from build123d import *

# Parameters (mm, degrees)
ESQUISSE1_R        = 2.5
ESQUISSE1_R_2      = 1.5
BOSS_EXTRU_1_DEPTH = 1.5
CONG_1_R           = 4


with BuildPart() as part:
    # Esquisse1 → Boss.-Extru.1 (new body)
    with BuildSketch(Plane.XY):
        Polygon((38, -20), (38, -32.5), (0, -32.5), (0, 32.5), (38, 32.5), (38, 20), (18, 20), (18, -20), align=None)
        with Locations((8, 25)):
            Circle(ESQUISSE1_R, mode=Mode.SUBTRACT)
        with Locations((23, 24)):
            Circle(ESQUISSE1_R_2, mode=Mode.SUBTRACT)
        with Locations(Location((33, 24, 0), (0, 0, 180))):
            Circle(ESQUISSE1_R_2, mode=Mode.SUBTRACT)
        with Locations((33, -24)):
            Circle(ESQUISSE1_R_2, mode=Mode.SUBTRACT)
        with Locations(Location((23, -24, 0), (0, 0, 180))):
            Circle(ESQUISSE1_R_2, mode=Mode.SUBTRACT)
        with Locations(Location((8, -25, 0), (0, 0, 180))):
            Circle(ESQUISSE1_R, mode=Mode.SUBTRACT)
    extrude(amount=BOSS_EXTRU_1_DEPTH)

    # Congé1
    cong_1_edges = [part.edges().sort_by_distance(p)[0] for p in [
        (38, -32.5, 0.75),
        (0, -32.5, 0.75),
        (0, 32.5, 0.75),
        (38, 32.5, 0.75),
    ]]
    fillet(cong_1_edges, radius=CONG_1_R)


solid = part.part
The listing builds one solid part. Answer for the finished solid, in the listing's coordinates (mm). A direction names the side the tool comes from. Coordinates: 2 decimals unless noted, no trailing zeros. Loops run counter-clockwise (first coordinate to the right, second up) from the corner with the lowest first, then second, coordinate; pieces in that order, holes last. Notation, with made-up numbers: (38.25, 63.5) -> (54.25, 63.5) arc R17 cw to (54.25, 79.5) -> close; hole circle Ø5 at (75, 2). An arc over 180 degrees is marked (long way). Write item = value, one per line. Start each with the question number.
1) A cutting plane is placed at A-A (x = 22.5). Give the vertices of the cut face in (y, z).
2) A cutting plane is placed at B-B (z = 0.3). Give the vertices of the cut face in (x, y), then the cut area to 3 significant figures.
3) A tool of negligible diameter and unlimited length cuts with its end or side. For faces 1 (the face through (31.89, -22.99, 0.74)), 2 (the face through (18, 0, 1)), from which of +Z, -Z, +X, -X, +Y, -Y can it reach the whole face along a straight path? Write none if from no direction.
4) A cutting plane is placed at C-C (x = 30.5). Give the vertices of the cut face in (y, z), then the cut area to 3 significant figures.
5) Straight lines are drawn through the part: line 1 (Y direction, x = 23, z = 1.15); line 2 (Y direction, x = 8, z = 1.1); line 3 (Y direction, x = 29, z = 0.85). For each, find the intervals that lie inside material, in ascending order. Write a range as from..to.
6) A cutting plane is placed at D-D (y = -9). Give the vertices of the cut face in (x, z).
7) The mould has two halves that part along Y. Classify faces 3 (the face through (15, 0, 0)), 4 (the face through (28, 20, 1)), 5 (the face through (1.203, -31.359, 0.76)): released by +Y, released by -Y, zero draft, split by the parting line, or undercut.
Responses:
q1.outline = (-32.5, 0) -> (-25.41, 0) -> (-25.41, 1.5) -> (-32.5, 1.5) -> close; (-22.59, 0) -> (-20, 0) -> (-20, 1.5) -> (-22.59, 1.5) -> close; (20, 0) -> (22.59, 0) -> (22.59, 1.5) -> (20, 1.5) -> close; (25.41, 0) -> (32.5, 0) -> (32.5, 1.5) -> (25.41, 1.5) -> close
q2.outline = (0, -28.5) arc R4 ccw to (4, -32.5) -> (34, -32.5) arc R4 ccw to (38, -28.5) -> (38, -20) -> (18, -20) -> (18, 20) -> (38, 20) -> (38, 28.5) arc R4 ccw to (34, 32.5) -> (4, 32.5) arc R4 ccw to (0, 28.5) -> close; hole circle Ø5 at (8, -25); hole circle Ø5 at (8, 25); hole circle Ø3 at (23, -24); hole circle Ø3 at (23, 24); hole circle Ø3 at (33, -24); hole circle Ø3 at (33, 24)
q2.area = 1,590 mm²
q3.face_1 = +Z, -Z
q3.face_2 = +Z, -Z, +X
q4.outline = (-32.5, 0) -> (-20, 0) -> (-20, 1.5) -> (-32.5, 1.5) -> close; (20, 0) -> (32.5, 0) -> (32.5, 1.5) -> (20, 1.5) -> close
q4.area = 37.5 mm²
q5.line_1 = -32.5..-25.5, -22.5..-20, 20..22.5, 25.5..32.5
q5.line_2 = -32.5..-27.5, -22.5..22.5, 27.5..32.5
q5.line_3 = -32.5..-20, 20..32.5
q6.outline = (0, 0) -> (18, 0) -> (18, 1.5) -> (0, 1.5) -> close
q7.face_3 = zero draft
q7.face_4 = undercut
q7.face_5 = released by -Y
